Part model, mm, in its own coordinate system. Face numbers are marked on the shaded views. Give positions to 0.01 mm unless a question says otherwise; leave off trailing zeros. Order: outer loops, then holes, each group sorted by start corner. A loop starts at its lowest first (then second) coordinate and runs counter-clockwise, first axis right, second up. Notation, with made-up numbers: (75, 41.5) -> (121, 41.5) arc R20 ccw to (121, 72.5) -> close; hole circle Ø6 at (77.25, 11.5). An arc over 180 degrees is marked (long way). Write item = value, one per line. Start each with the question number.
Item 1: Flat gauge pins, fed straight in: P1, Ø6, axis at x = -0.5, y = -1, coming from the -Z side; P2, Ø3, axis at y = 3, z = 2, coming from the +X side. Where does each tip first touch, or does it go through?
Item 2: Drill centre lines: line 1 along Y through (x, z) = (0, 3.6); line 2 along X through (y, z) = (1, 1.3); line 3 along X through (y, z) = (-2.5, 2.8). Where is each one in solid material? Low to high.
Item 3: Pull direction X, two halves, no side cores. Call the marked faces 1, 2, 3 and 4: +X half, -X half, draft (parallel to the pull), parting line (faces both ways), or undercut.
Item 4: Band-saw the part on B-B on z = 3.7. Write the cut outline in (x, y), plus the area to 3 significant figures.
Item 5: Band-saw the part on A-A on x = 0. Write the cut outline in (y, z).
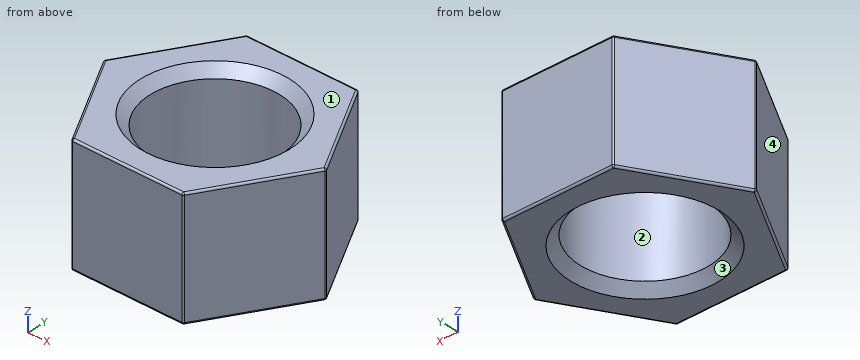
```python
from build123d import *

# Parameters (mm, degrees)
SKETCH1_R           = 3.3
BOSS_EXTRUDE1_DEPTH = 6
FILLET1_R           = 0.1
CHAMFER1_SIZE       = 0.5


with BuildPart() as part:
    # Sketch1 → Boss-Extrude1 (new body)
    with BuildSketch(Plane.XY):
        Polygon((-2.886751346, -5), (2.886751346, -5), (5.773502692, 0), (2.886751346, 5), (-2.886751346, 5), (-5.773502692, 0), align=None)
        Circle(SKETCH1_R, mode=Mode.SUBTRACT)
    extrude(amount=BOSS_EXTRUDE1_DEPTH)

    # Fillet1
    fillet1_edges = [part.edges().sort_by_distance(p)[0] for p in [
        (-5.773502692, 0, 3),
        (-2.886751346, 5, 3),
        (2.886751346, 5, 3),
        (5.773502692, 0, 3),
        (2.886751346, -5, 3),
        (-2.886751346, -5, 3),
        (4.330127019, -2.5, 6),
        (4.330127019, 2.5, 6),
        (0, 5, 6),
        (-4.330127019, 2.5, 6),
        (-4.330127019, -2.5, 6),
        (-4.330127019, 2.5, 0),
        (0, 5, 0),
        (4.330127019, 2.5, 0),
        (4.330127019, -2.5, 0),
        (0, -5, 0),
        (-4.330127019, -2.5, 0),
        (0, -5, 6),
    ]]
    fillet(fillet1_edges, radius=FILLET1_R)

    # Chamfer1
    chamfer1_edges = [part.edges().sort_by_distance(p)[0] for p in [
        (-3.3, 0, 0),
        (-3.3, 0, 6),
    ]]
    chamfer(chamfer1_edges, length=CHAMFER1_SIZE)


solid = part.part
```
Values found:
q1.P1 = 0
q1.P2 = 4.91
q2.line_1 = -5 to -3.3, 3.3 to 5
q2.line_2 = -5.2 to -3.14, 3.14 to 5.2
q2.line_3 = -4.33 to -2.15, 2.15 to 4.33
q3.face_1 = draft
q3.face_2 = undercut
q3.face_3 = undercut
q3.face_4 = -X half
q4.outline = (-5.74, -0.05) -> (-2.92, -4.95) arc R0.1 ccw to (-2.83, -5) -> (2.83, -5) arc R0.1 ccw to (2.92, -4.95) -> (5.74, -0.05) arc R0.1 ccw to (5.74, 0.05) -> (2.92, 4.95) arc R0.1 ccw to (2.83, 5) -> (-2.83, 5) arc R0.1 ccw to (-2.92, 4.95) -> (-5.74, 0.05) arc R0.1 ccw to start; hole circle Ø6.6 at (0, 0)
q4.area = 52.4 mm^2
q5.outline = (-5, 0.1) arc R0.1 ccw to (-4.9, 0) -> (-3.8, 0) -> (-3.3, 0.5) -> (-3.3, 5.5) -> (-3.8, 6) -> (-4.9, 6) arc R0.1 ccw to (-5, 5.9) -> close; (3.3, 0.5) -> (3.8, 0) -> (4.9, 0) arc R0.1 ccw to (5, 0.1) -> (5, 5.9) arc R0.1 ccw to (4.9, 6) -> (3.8, 6) -> (3.3, 5.5) -> close
